Input: part model. Units: mm. Frame: model coordinates. A direction names the side the tool comes from. Coordinates: 2 decimals unless noted, no trailing zeros. Loops run counter-clockwise (first coordinate to the right, second up) from the corner with the lowest first, then second, coordinate; pieces in that order, holes last.
Item 1: Contact query for flat-ended pins moving along their axis: P1, Ø1.2, axis at x = -100.5, y = 1.5, coming from the -Z side; P2, Ø10.5, axis at x = -92, y = 13.5, coming from the +Z side; P3, Ø0.6, axis at x = -125, z = 0, coming from the -Y side. Output: stop coordinate, or through.
Item 2: Pull-direction query (X, two-part tool) for faces 6 (the flat face through (2, -1.1, -9)), 7 (the flat face through (-124.612, -2, -22)), 8 (the flat face through (125.188, 0, -22)), 9 (the flat face through (100, 9, -27.968)); classes: released by +X, released by -X, zero draft, split by the parting line, or undercut.
Item 3: Section B-B on y = 8.5. Return loops of the section in (x, z), and give its area (3 significant figures).
Item 4: Section D-D on x = -93. Return loops of the section in (y, z).
Item 5: Section C-C on x = 23. Return loops of the section in (y, z).
Item 6: Ray query, line 1 along X through (y, z) = (0.25, 23); line 2 along Y through (x, z) = (-26.5, -6.5); line 3 along X through (y, z) = (-0.5, 0.5). Return the intervals inside material, ascending.
Item 7: Reachability of faces 1 (the flat face through (93.32, 11.03, -26.39)), 2 (the flat face through (2, -1, -70.968)), 3 (the flat face through (-99, 9, -27.968)), 4 (the flat face through (-99, 9, -24.768)), 5 (the flat face through (2, -1, 29.032)) from +Z, -Z, +X, -X, +Y, -Y: full face, straight path, thin tool, end or side. Return the list, or none.
Item 8: Section A-A on z = 19.5. Return loops of the section in (x, y).
```python
from build123d import *

# Parameters (mm, degrees)
F0_W      = 249.8
F0_H      = 100
F1_DEPTH  = 4
F4_W      = 20
F4_H      = 10
F5_DEPTH  = 4
F6_W      = 48
F6_H      = 65
F7_DEPTH  = 4
F8_W      = 20
F8_H      = 10
F9_DEPTH  = 4
F10_DEPTH = 1.1
F11_W     = 20
F11_H     = 3.2
F12_DEPTH = 13
F13_SIZE  = 12.1
F14_R     = 2


# Not quite as in the source:
# - a feature names something its author has since deleted; it is built from what else it names


with BuildPart() as f1:
    # F0 (on Front) → F1 (new body)
    with BuildSketch(Plane.XZ):
        with Locations((0.2878084779, -20.9680776408)):
            Rectangle(F0_W, F0_H)
    extrude(amount=F1_DEPTH)

    # F4 (on face) → F5 (join)
    with BuildSketch(Plane(origin=(0, 0, 0), x_dir=(-1, 0, 0), z_dir=(0, 1, 0))):
        with Locations((-115.1878084779, -65.9680776408)):
            Rectangle(F4_W, F4_H)
        with Locations((114.6121915221, -65.9680776408)):
            Rectangle(F4_W, F4_H)
    extrude(amount=F5_DEPTH)

    # F6 (on face) → F7 (join)
    with BuildSketch(Plane(origin=(0, 0, 0), x_dir=(-1, 0, 0), z_dir=(0, 1, 0))):
        with Locations((-101.1878084779, -3.4680776408)):
            Rectangle(F6_W, F6_H)
        with Locations((101.1878084779, -3.4680776408)):
            Rectangle(F6_W, F6_H)
    extrude(amount=F7_DEPTH)

    # F8 (on face) → F9 (join)
    with BuildSketch(Plane(origin=(0, 0, 0), x_dir=(-1, 0, 0), z_dir=(0, 1, 0))):
        with Locations((114.6121915221, -65.9680776408)):
            Rectangle(F8_W, F8_H)
    extrude(amount=F9_DEPTH)

    # F2 (on face) → F10 (cut)
    with BuildSketch(Plane(origin=(0, 0, 0), x_dir=(-1, 0, 0), z_dir=(0, 1, 0))):
        Polygon((41.6121915221, 16.0319223592), (-44.3878084779, 16.0319223592), (-44.3878084779, 6.0319223592), (-44.3878084779, -23.9680776408), (-44.3878084779, -33.9680776408), (41.6121915221, -33.9680776408), (41.6121915221, 6.0319223592), align=None)
    extrude(amount=-F10_DEPTH, mode=Mode.SUBTRACT)

    # F11 (on face) → F12 (join)
    with BuildSketch(Plane(origin=(0, 4, 0), x_dir=(-1, 0, 0), z_dir=(0, 1, 0))):
        with Locations((-97.1878084779, -26.3680776408)):
            Rectangle(F11_W, F11_H)
        with Locations((97.1878084779, -26.3680776408)):
            Rectangle(F11_W, F11_H)
    extrude(amount=F12_DEPTH)

    # F13
    f13_edges = [f1.edges().sort_by_distance(p)[0] for p in [
        (87.187808, 17, -26.368078),
        (-87.187808, 17, -26.368078),
    ]]
    chamfer(f13_edges, length=F13_SIZE)

    # F14
    f14_edges = [f1.edges().sort_by_distance(p)[0] for p in [
        (107.187808, 17, -26.368078),
        (-107.187808, 17, -26.368078),
    ]]
    fillet(f14_edges, radius=F14_R)


solid = f1.part
```
Results found:
1. P1: stops at z = -35.97
1. P2: stops at z = -24.77
1. P3: stops at y = 0
2. face 6: undercut
2. face 7: released by -X
2. face 8: released by +X
2. face 9: zero draft
3. outline: (-107.19, -27.97) - (-90.79, -27.97) - (-90.79, -24.77) - (-107.19, -24.77) - close; (90.79, -27.97) - (107.19, -27.97) - (107.19, -24.77) - (90.79, -24.77) - close
3. area: 105 mm2
4. outline: (-4, -70.97) - (0, -70.97) - (0, -35.97) - (4, -35.97) - (4, -27.97) - (10.71, -27.97) - (10.71, -24.77) - (4, -24.77) - (4, 29.03) - (-4, 29.03) - close
5. outline: (-4, -70.97) - (0, -70.97) - (0, -33.97) - (-1.1, -33.97) - (-1.1, 16.03) - (0, 16.03) - (0, 29.03) - (-4, 29.03) - close
6. line 1: x = -125.19 to -77.19, 77.19 to 125.19
6. line 2: y = -4 to -1.1
6. line 3: x = -124.61 to -41.61, 44.39 to 125.19
7. face 1: +Z, -Z, +Y
7. face 2: -Z, +X, -X, +Y, -Y
7. face 3: -Z, +X, -X, +Y
7. face 4: +Z, +X, -X, +Y
7. face 5: +Z, +X, -X, +Y, -Y
8. outline: (-125.19, 0) - (-124.61, 0) - (-124.61, -4) - (125.19, -4) - (125.19, 4) - (77.19, 4) - (77.19, 0) - (-77.19, 0) - (-77.19, 4) - (-125.19, 4) - close
